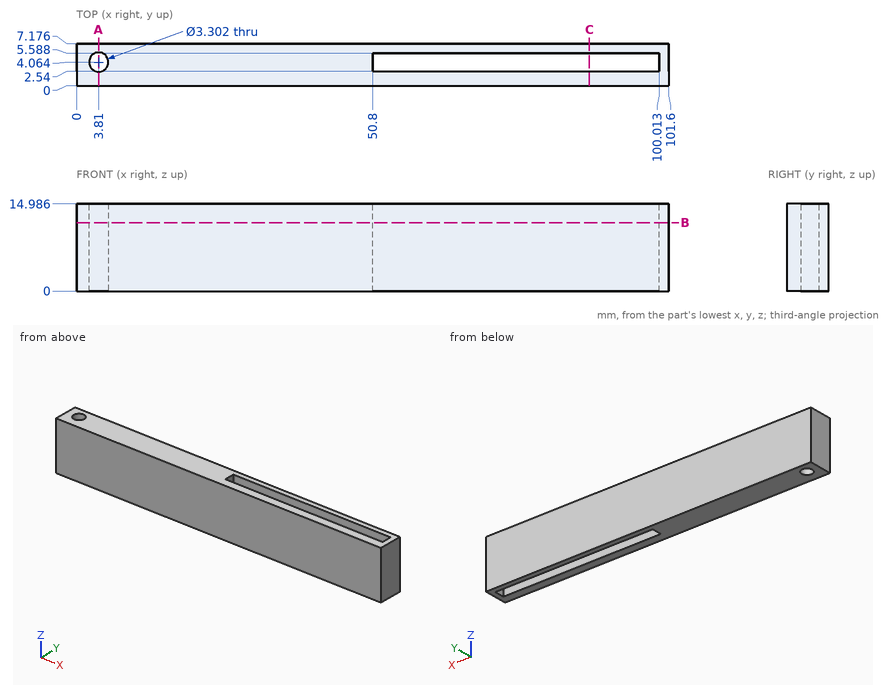
Design review of the part shown in the three views and the two pictorial views. Dimensions are in mm from the part's minimum x, y and z. Round coordinates to 2 decimals unless told otherwise and drop trailing zeros. Write each loop counter-clockwise with the first axis right and the second up, starting at its lowest first coordinate (ties: lowest second). Pieces come first, ordered by that corner, then holes. Notation, with made-up numbers: M -39,49 L -1,49 A22 ccw -1,69 Z; hole C -33,81.25 d8. An arc over 180 degrees is marked long. One line per item, written item: value. Start each with the question number.
1. Take a section at B-B on z = 11.75. State how many separate pieces and enclosed holes the cut face has.
2. Take a section at A-A on x = 3.81. State the section outline as (y, z) points (1 decimal).
3. To check wall thickness, follow probe 1 along Y at (x, z) = (3.81, 7.75) (1 decimal); probe 2 along X at (y, z) = (4, 6.75); probe 3 along X at (y, z) = (5, 13.75). State the ranges of each line that lie inside material, in increasing order. Write a range as from..to.
4. Take a section at C-C on x = 88. State the section outline as (y, z) points (1 decimal).
5. Clearance check with a flat-ended pin moving along its axis: P1, Ø1, axis at x = 76, y = 5, coming from the +Z side. State where the tip first meets the part, or that it passes through.
Computed:
1. separate pieces: 1
1. enclosed holes: 2
2. outline: M 0,0 L 2.4,0 L 2.4,15 L 0,15 Z; M 5.7,0 L 7.2,0 L 7.2,15 L 5.7,15 Z
3. probe 1: y = 0..2.4, 5.7..7.2
3. probe 2: x = 0..2.16, 5.46..50.8, 100.01..101.6
3. probe 3: x = 0..2.45, 5.17..50.8, 100.01..101.6
4. outline: M 0,0 L 2.5,0 L 2.5,15 L 0,15 Z; M 5.6,0 L 7.2,0 L 7.2,15 L 5.6,15 Z
5. P1: passes through
